Part model, mm, in its own coordinate system. A direction names the side the tool comes from. Round coordinates to 2 decimals unless told otherwise and drop trailing zeros. Loops run counter-clockwise (first coordinate to the right, second up) from the corner with the lowest first, then second, coordinate; pieces in that order, holes last. Notation, with made-up numbers: (58.5, -18) -> (115.5, -18) arc R18 ccw to (115.5, 14) -> close; hole circle Ø8 at (63.5, -9). An arc over 180 degrees is marked (long way). Answer as CSV lines item,"result".
from build123d import *

# Parameters (mm, degrees)
F0_W          = 22
F0_H          = 8
F0_W_2        = 21.6
F0_H_2        = 7.6
F0_W_3        = 17.6
F0_H_3        = 3.6
F1_DEPTH      = 2
F2_DEPTH      = 4
F3_R          = 2.5
F4_DEPTH      = 10
F4_DEPTH_BACK = 10
F5_R          = 0.75
F6_DEPTH      = 24.801
F6_DEPTH_BACK = 3.201


with BuildPart() as f1:
    # F0 (on Top) → F1 (new body)
    with BuildSketch(Plane.XY):
        with BuildLine():
            Line((17.5520906094, 3.2524078637), (17.5520906094, 7.2524078637))
            ThreePointArc((17.5520906094, 7.2524078637), (16.0876245154, 10.7879417697), (12.5520906094, 12.2524078637))
            Line((12.5520906094, 12.2524078637), (-5.4479093906, 12.2524078637))
            ThreePointArc((-5.4479093906, 12.2524078637), (-8.9834432965, 10.7879417697), (-10.4479093906, 7.2524078637))
            Line((-10.4479093906, 7.2524078637), (-10.4479093906, 3.2524078637))
            ThreePointArc((-10.4479093906, 3.2524078637), (-8.9834432965, -0.2831260422), (-5.4479093906, -1.7475921363))
            Line((-5.4479093906, -1.7475921363), (12.5520906094, -1.7475921363))
            ThreePointArc((12.5520906094, -1.7475921363), (16.0876245154, -0.2831260422), (17.5520906094, 3.2524078637))
        make_face()
        with Locations((3.5520906094, 5.2524078637)):
            Rectangle(F0_W, F0_H, mode=Mode.SUBTRACT)
        with Locations((3.5520906094, 5.2524078637)):
            Rectangle(F0_W, F0_H)
        with Locations((3.5520906094, 5.2524078637)):
            Rectangle(F0_W_2, F0_H_2, mode=Mode.SUBTRACT)
        with Locations((3.5520906094, 5.2524078637)):
            Rectangle(F0_W_2, F0_H_2)
        with Locations((3.5520906094, 5.2524078637)):
            Rectangle(F0_W_3, F0_H_3, mode=Mode.SUBTRACT)
        with Locations((3.5520906094, 5.2524078637)):
            Rectangle(F0_W_3, F0_H_3)
    extrude(amount=-F1_DEPTH)

    # F0 (on Top) → F2 (join)
    with BuildSketch(Plane.XY):
        with Locations((3.5520906094, 5.2524078637)):
            Rectangle(F0_W_2, F0_H_2)
        with Locations((3.5520906094, 5.2524078637)):
            Rectangle(F0_W_3, F0_H_3, mode=Mode.SUBTRACT)
    extrude(amount=F2_DEPTH)

    # F3 (on face) → F4 (cut, two sides)
    with BuildSketch(Plane(origin=(0, 0, -2), x_dir=(1, 0, 0), z_dir=(0, 0, -1))) as f4_sk:
        with Locations((3.5520906094, -5.2524078637)):
            Circle(F3_R)
    extrude(amount=-F4_DEPTH, mode=Mode.SUBTRACT)
    extrude(f4_sk.sketch, amount=F4_DEPTH_BACK, mode=Mode.SUBTRACT)

    # F5 (on face) → F6 (cut, two sides)
    with BuildSketch(Plane(origin=(-7.2479093906, 0, 0), x_dir=(0, -1, 0), z_dir=(-1, 0, 0))) as f6_sk:
        with Locations((-5.2524078637, 2)):
            Circle(F5_R)
    extrude(amount=-F6_DEPTH, mode=Mode.SUBTRACT)
    extrude(f6_sk.sketch, amount=F6_DEPTH_BACK, mode=Mode.SUBTRACT)


solid = f1.part
Q1. Saw through at A-A, the plane z = 3.55. Write the cut outline in (x, y).
Geometry results:
outline,"(-7.25, 1.45) -> (14.35, 1.45) -> (14.35, 9.05) -> (-7.25, 9.05) -> close; hole (-5.25, 3.45) -> (1.82, 3.45) arc R2.5 ccw to (5.29, 3.45) -> (12.35, 3.45) -> (12.35, 7.05) -> (5.29, 7.05) arc R2.5 ccw to (1.82, 7.05) -> (-5.25, 7.05) -> close"
Q2. Drill centre lines: line 1 along Y through (x, z) = (8.25, 0.9); line 2 along X through (y, z) = (2.5, 1.5); line 3 along Z through (x, y) = (15, 11.5). Where is each one in solid material? Low to high.
Geometry results:
line 1,"1.45 to 3.45, 7.05 to 9.05"
line 2,"-7.25 to 14.35"
line 3,"-2 to 0"
Q3. Drop flat-ended pins along their axis: P1, Ø2, axis at y = 7.5, z = 1.5, coming from the -X side; P2, Ø3, axis at y = 6, z = 2.5, coming from the +X side; P3, Ø2, axis at x = 7, z = 3, coming from the -Y side. Give the stop position or say it passes through.
Geometry results:
P1,"x = -7.25"
P2,"x = 14.35"
P3,"y = 1.45"
Q4. Saw through at C-C, the plane z = 2. Write the cut outline in (x, y), then the cut area to 3 significant figures.
Geometry results:
outline,"(-7.25, 1.45) -> (14.35, 1.45) -> (14.35, 4.5) -> (12.35, 4.5) -> (12.35, 3.45) -> (5.29, 3.45) arc R2.5 cw to (1.82, 3.45) -> (-5.25, 3.45) -> (-5.25, 4.5) -> (-7.25, 4.5) -> close; (-7.25, 6) -> (-5.25, 6) -> (-5.25, 7.05) -> (1.82, 7.05) arc R2.5 cw to (5.29, 7.05) -> (12.35, 7.05) -> (12.35, 6) -> (14.35, 6) -> (14.35, 9.05) -> (-7.25, 9.05) -> close"
area,"91.5 mm2"
Q5. Saw through at D-D, the plane x = 6.75. Write the cut outline in (y, z), then the cut area to 3 significant figures.
Geometry results:
outline,"(-1.75, -2) -> (12.25, -2) -> (12.25, 0) -> (9.05, 0) -> (9.05, 4) -> (7.05, 4) -> (7.05, 0) -> (3.45, 0) -> (3.45, 4) -> (1.45, 4) -> (1.45, 0) -> (-1.75, 0) -> close"
area,"44.0 mm2"
Q6. Which spindle directions (+Z, -Z, +X, -X, +Y, -Y) get a long thin tool onto all of the face, cutting with end or side? Do faces 4 (the face through (16.126, 10.749, -0.986)), 5 (the face through (-7.248, 4, 2)), 6 (the face through (-2, 7.052, 2)), 7 (the face through (3, 1.452, 2)). Say none if no direction does.
Geometry results:
face 4,"+Z, -Z, +X, +Y"
face 5,"+Z, -X, +Y, -Y"
face 6,"+Z"
face 7,"+Z, +X, -X, -Y"
Q7. Saw through at B-B, the plane x = 3. Write the cut outline in (y, z), then the cut area to 3 significant figures.
Geometry results:
outline,"(-1.75, -2) -> (2.81, -2) -> (2.81, 4) -> (1.45, 4) -> (1.45, 0) -> (-1.75, 0) -> close; (7.69, -2) -> (12.25, -2) -> (12.25, 0) -> (9.05, 0) -> (9.05, 4) -> (7.69, 4) -> close"
area,"29.1 mm2"
Q8. Two-plate mould, pull along Y, no slides. Class faces 1 (the face through (3, -1.748, -1)), 2 (the face through (3, 8, 4)), 3 (the face through (-2, 3.452, 2)): pulls with the +Y half, pulls with the -Y half, needs draft (parallel to the pull), parting line crosses it, or undercut.
Geometry results:
face 1,"pulls with the -Y half"
face 2,"needs draft"
face 3,"undercut"
